Design review of the part built by this model. Coordinates are the model's own, in mm. A direction names the side the tool comes from. Coordinates: 2 decimals unless noted, no trailing zeros. Loops run counter-clockwise (first coordinate to the right, second up) from the corner with the lowest first, then second, coordinate; pieces in that order, holes last. Notation, with made-up numbers: (25, -18.5) -> (30, -18.5) arc R14 ccw to (30, -2.5) -> close; hole circle Ø6 at (34, 6). An arc over 180 degrees is marked (long way). Use CSV: the item, a comma, the result in double quotes.
```python
from build123d import *

# Parameters (mm, degrees)
SKETCH1_W           = 67
SKETCH1_H           = 155
SKETCH1_W_2         = 160
SKETCH1_H_2         = 110
SKETCH1_W_3         = 18.62
SKETCH1_H_3         = 29.1
BOSS_EXTRUDE1_DEPTH = 5
SKETCH4_W           = 100
SKETCH4_H           = 2
BOSS_EXTRUDE2_DEPTH = 10
SKETCH9_W           = 0.845761127
SKETCH9_H           = 22.5
BOSS_EXTRUDE4_DEPTH = 5
BOSS_EXTRUDE3_DEPTH = 5
SKETCH7_R           = 2.05
CUT_EXTRUDE2_DEPTH  = 10
SKETCH6_R           = 2.05
CUT_EXTRUDE1_DEPTH  = 227.055622359
SKETCH10_R          = 2.05
CUT_EXTRUDE4_DEPTH  = 10
FILLET1_R           = 0.3
SKETCH16_R          = 2.05
CUT_EXTRUDE5_DEPTH  = 251.551680098


with BuildPart() as part:
    # Sketch1 → Boss-Extrude1 (new body)
    with BuildSketch(Plane(origin=(0, 0, 0), x_dir=(1, 0, 0), z_dir=(0, 1, 0))):
        Rectangle(SKETCH1_W, SKETCH1_H)
        with Locations((-113.5, 0)):
            Rectangle(SKETCH1_W_2, SKETCH1_H_2)
        with Locations((-202.81, 0)):
            Rectangle(SKETCH1_W_3, SKETCH1_H_3)
    extrude(amount=BOSS_EXTRUDE1_DEPTH)

    # Sketch4 → Boss-Extrude2 (add)
    with BuildSketch(Plane(origin=(0, 5, 0), x_dir=(1, 0, 0), z_dir=(0, 1, 0))):
        with Locations((-143.5, -54)):
            Rectangle(SKETCH4_W, SKETCH4_H)
        with Locations((-143.5, 54)):
            Rectangle(SKETCH4_W, SKETCH4_H)
    extrude(amount=BOSS_EXTRUDE2_DEPTH)

    # Sketch9 → Boss-Extrude4 (add)
    with BuildSketch(Plane(origin=(0, 5, 0), x_dir=(1, 0, 0), z_dir=(0, 1, 0))):
        with Locations((-33.922880564, -66.25)):
            Rectangle(SKETCH9_W, SKETCH9_H)
        with Locations((-33.922880564, 66.25)):
            Rectangle(SKETCH9_W, SKETCH9_H)
    extrude(amount=-BOSS_EXTRUDE4_DEPTH)

    # Sketch5 → Boss-Extrude3 (add)
    with BuildSketch(Plane(origin=(0, 5, 0), x_dir=(1, 0, 0), z_dir=(0, 1, 0))):
        Polygon((-178, 27), (-172.5, 27), (-172.5, 34.2), (-183.5, 34.2), (-183.5, 19.3), (-178, 19.3), align=None)
        Polygon((-178, -27.15), (-172.5, -27.15), (-172.5, -34.35), (-183.5, -34.35), (-183.5, -19.45), (-178, -19.45), align=None)
        Polygon((-13.85, 27), (-13.85, 19.3), (-8.35, 19.3), (-8.35, 34.2), (-19.35, 34.2), (-19.35, 27), align=None)
        Polygon((-19.35, -27.15), (-19.35, -34.35), (-8.35, -34.35), (-8.35, -19.45), (-13.85, -19.45), (-13.85, -27.15), align=None)
    extrude(amount=BOSS_EXTRUDE3_DEPTH)

    # Sketch7 → Cut-Extrude2 (cut)
    with BuildSketch(Plane(origin=(0, 5, 0), x_dir=(1, 0, 0), z_dir=(0, 1, 0))):
        with Locations(Location((-207.12, 10.268043156, 0), (0, 0, 270))):
            Circle(SKETCH7_R)
        with Locations(Location((-207.12, -9.741956844, 0), (0, 0, 270))):
            Circle(SKETCH7_R)
    extrude(amount=-CUT_EXTRUDE2_DEPTH, mode=Mode.SUBTRACT)

    # Sketch6 → Cut-Extrude1 (cut, through all)
    with BuildSketch(Plane(origin=(0, 5, 0), x_dir=(1, 0, 0), z_dir=(0, 1, 0))):
        with Locations(Location((-85.880982052, -48, 0), (0, 0, 270))):
            Circle(SKETCH6_R)
        with Locations(Location((-57.380982052, -48, 0), (0, 0, 270))):
            Circle(SKETCH6_R)
        with Locations(Location((-57.380982052, 48, 0), (0, 0, 90))):
            Circle(SKETCH6_R)
        with Locations(Location((-85.880982052, 48, 0), (0, 0, 90))):
            Circle(SKETCH6_R)
    extrude(amount=-CUT_EXTRUDE1_DEPTH, mode=Mode.SUBTRACT)

    # Sketch10 → Cut-Extrude4 (cut)
    with BuildSketch(Plane(origin=(0, 5, 0), x_dir=(1, 0, 0), z_dir=(0, 1, 0))):
        with Locations(Location((-183.5, 44.599757133, 0), (0, 0, 270))):
            Circle(SKETCH10_R)
        with Locations(Location((-137.5, 44.599757133, 0), (0, 0, 270))):
            Circle(SKETCH10_R)
        with Locations(Location((-183.5, -43.400242867, 0), (0, 0, 270))):
            Circle(SKETCH10_R)
        with Locations(Location((-137.5, -43.400242867, 0), (0, 0, 270))):
            Circle(SKETCH10_R)
    extrude(amount=-CUT_EXTRUDE4_DEPTH, mode=Mode.SUBTRACT)

    # Fillet1
    fillet1_edges = [part.edges().sort_by_distance(p)[0] for p in [
        (-34.345761127, 2.5, 55),
        (-34.345761127, 2.5, -55),
    ]]
    fillet(fillet1_edges, radius=FILLET1_R)

    # Sketch16 → Cut-Extrude5 (cut, through all)
    with BuildSketch(Plane.XY.offset(55)):
        with Locations((-140.228178999, 10)):
            Circle(SKETCH16_R)
        with Locations((-125.228178999, 10)):
            Circle(SKETCH16_R)
        with Locations((-110.228178999, 10)):
            Circle(SKETCH16_R)
        with Locations((-155.228178999, 10)):
            Circle(SKETCH16_R)
        with Locations((-170.228178999, 10)):
            Circle(SKETCH16_R)
        with Locations((-185.228178999, 10)):
            Circle(SKETCH16_R)
    extrude(amount=-CUT_EXTRUDE5_DEPTH, mode=Mode.SUBTRACT)


solid = part.part
```
Item 1: Add section A-A (x = -120). Give the boundary of the cut face in (y, z), then the cut area to 3 significant figures.
Checked values:
outline,"(0, -55) -> (15, -55) -> (15, -53) -> (5, -53) -> (5, 53) -> (15, 53) -> (15, 55) -> (0, 55) -> close"
area,"590 mm^2"
Item 2: Draft analysis for pull direction Z (two halves, no side actions). For faces 4 (the face through (-1, 3, 77.5)), 5 (the face through (-8.35, 7, -27)), 6 (the face through (-172.5, 7, -31)), state which applies: pulls with the +Z half, pulls with the -Z half, needs draft (parallel to the pull), parting line crosses it, or undercut.
Checked values:
face 4,"pulls with the +Z half"
face 5,"needs draft"
face 6,"undercut"
Item 3: Add section B-B (z = 29.5). Give the boundary of the cut face in (x, y), then the cut area to 3 significant figures.
Checked values:
outline,"(-193.5, 0) -> (33.5, 0) -> (33.5, 5) -> (-8.35, 5) -> (-8.35, 10) -> (-19.35, 10) -> (-19.35, 5) -> (-172.5, 5) -> (-172.5, 10) -> (-183.18, 10) arc R2.05 cw to (-183.5, 8.9) -> (-183.5, 5) -> (-193.5, 5) -> close"
area,"1,240 mm^2"
Item 4: Add section D-D (x = -62). Give the boundary of the cut face in (y, z).
Checked values:
outline,"(0, -55) -> (5, -55) -> (5, 55) -> (0, 55) -> close"
Item 5: Machinability: for faces 1 (the face through (-193.5, 4, -36)), 2 (the face through (-11, 7, 19.45)), 3 (the face through (-17, 7, -27)), which of the approach directions +Z, -Z, +X, -X, +Y, -Y give a long, thin tool a straight path to every point of the face, cutting with its end or side? Answer none if there is none.
Checked values:
face 1,"-Z, -X, +Y, -Y"
face 2,"+X, -X, +Y"
face 3,"+Y"
Item 6: To check wall thickness, follow line 1 along X through (y, z) = (3.05, -48); line 2 along Z through (x, y) = (-139.5, 7.5); line 3 along Z through (x, y) = (-12.5, 8.25). State the ranges of each line that lie inside material, in increasing order.
Checked values:
line 1,"-193.5 to -87.93, -83.83 to -59.43, -55.33 to 33.5"
line 2,"-55 to -53, 53 to 55"
line 3,"-34.2 to -19.3, 19.45 to 34.35"
Item 7: Clearance check with flat-ended pins moving along their axes: pin 1 (1.5 mm diameter, centred on y = 6.5, z = -31.5, fed in from -X); pin 2 (4.5 mm diameter, centred on x = -183.5, z = -44.6, fed in from +Y); pin 3 (4 mm diameter, centred on y = 2, z = 53, fed in from -X). State where each tip first meets the part, or that it passes through.
Checked values:
pin 1,"x = -183.5"
pin 2,"y = 5"
pin 3,"x = -193.5"
Item 8: Add section C-C (z = 58.5). Give the boundary of the cut face in (x, y).
Checked values:
outline,"(-34.35, 0) -> (33.5, 0) -> (33.5, 5) -> (-34.35, 5) -> close"
